Build history of the part. All positions in model axes, mm. Face numbers are marked on the shaded views. A direction names the side the tool comes from. Give positions to 0.01 mm unless a question says otherwise; leave off trailing zeros. Order: outer loops, then holes, each group sorted by start corner. A loop starts at its lowest first (then second) coordinate and runs counter-clockwise, first axis right, second up. Notation, with made-up numbers: (30.5, 13.25) - (81.5, 13.25) arc R16 cw to (81.5, 21.25) - close; hole circle Ø8 at (76.5, 73.5). An arc over 180 degrees is marked (long way). One line per item, written item: value.
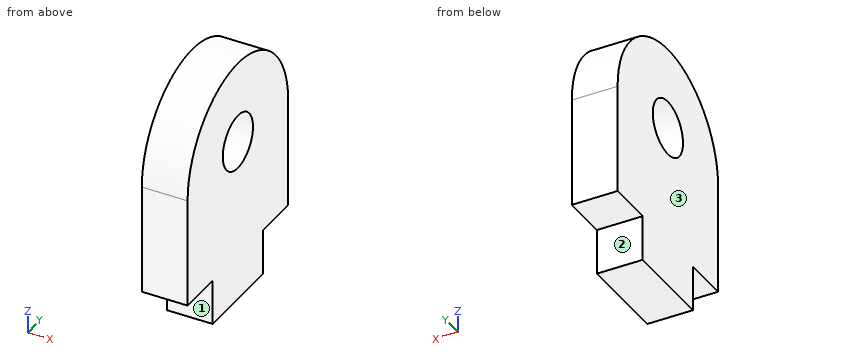
```python
from build123d import *

# Parameters (mm, degrees)
SKETCH1_R           = 3
BOSS_EXTRUDE1_DEPTH = 2.5
FILLET1_RADIUS      = 10
FILLET1_LENGTH      = 5


with BuildPart() as part:
    # Sketch1 → Boss-Extrude1 (new, symmetric)
    with BuildSketch(Plane.YZ):
        Polygon((-5, 0), (5, 0), (5, 5), (10, 5), (10, 27), (-10, 27), (-10, 5), (-5, 5), align=None)
        with Locations(Location((0, 18, 0), (0, 0, 270))):
            Circle(SKETCH1_R, mode=Mode.SUBTRACT)
    extrude(amount=BOSS_EXTRUDE1_DEPTH, both=True)

    # Fillet1: full round fillet: the end face becomes a half cylinder, R = half its width
    fillet1_face = Plane((0, 0, 27), x_dir=(-1, 0, 0), z_dir=(0, 0, 1))  # on the end face: x along it, z out of the body
    fillet1_slab = fillet1_face.offset(-FILLET1_RADIUS / 2) * Box(FILLET1_LENGTH, 2 * FILLET1_RADIUS, FILLET1_RADIUS, mode=Mode.PRIVATE)  # the body's end, R deep
    fillet1_round = Plane((0, 0, 17), x_dir=(0, 0, 1), z_dir=(-1, 0, 0)) * Cylinder(FILLET1_RADIUS, FILLET1_LENGTH, mode=Mode.PRIVATE)  # its axis R under the face
    add(fillet1_slab - fillet1_round, mode=Mode.SUBTRACT)


solid = part.part
```
(1) Slice it at D-D, the plane z = 25. Give the cut face in (x, y), and give its area (3 significant figures).
Completed:
outline: (-2.5, -6) - (2.5, -6) - (2.5, 6) - (-2.5, 6) - close
area: 60.0 mm²
(2) Slice it at C-C, the plane z = 18. Give the cut face in (x, y).
Completed:
outline: (-2.5, -9.95) - (2.5, -9.95) - (2.5, -3) - (-2.5, -3) - close; (-2.5, 3) - (2.5, 3) - (2.5, 9.95) - (-2.5, 9.95) - close
(3) Slice it at B-B, the plane x = 0.4. Give the cut face in (y, z), and give its area (3 significant figures).
Completed:
outline: (-10, 5) - (-5, 5) - (-5, 0) - (5, 0) - (5, 5) - (10, 5) - (10, 17) arc R10 ccw to (-10, 17) - close; hole circle Ø6 at (0, 18)
area: 419 mm²
(4) Pin check, flat tips, straight feed: P1, Ø1.5, axis at x = 1, z = 1.5, coming from the -Y side; P2, Ø3, axis at x = -0.5, z = 23.5, coming from the -Y side; P3, Ø2, axis at x = 1, y = -2, coming from the -Z side. Stop position of each tip, or through.
Completed:
P1: y = -5
P2: y = -8.66
P3: z = 0
(5) Drill centre lines: line 1 (Z direction, x = -2, y = 1.75); line 2 (Y direction, x = -1.2, z = 18); line 3 (Y direction, x = -1.65, z = 24.5). Where is each one in solid material? Low to high.
Completed:
line 1: 0 to 15.56, 20.44 to 26.85
line 2: -9.95 to -3, 3 to 9.95
line 3: -6.61 to 6.61
(6) 3-axis set-ups, long thin cutter, end or side, ignore diameter. For the marked faces 1, 2 and 3: which of +Z, -Z, +X, -X, +Y, -Y reach the whole face in a straight line?
Completed:
face 1: -Z, +X, -X, -Y
face 2: -Z, +X, -X, +Y
face 3: +Z, -Z, -X, +Y, -Y
(7) Slice it at A-A, the plane y = 0. Give the cut face in (x, z).
Completed:
outline: (-2.5, 0) - (2.5, 0) - (2.5, 15) - (-2.5, 15) - close; (-2.5, 21) - (2.5, 21) - (2.5, 27) - (-2.5, 27) - close
